Here's how the part is built. I have some questions about the finished solid (model axes, mm). A direction names the side the tool comes from. Round coordinates to 2 decimals unless told otherwise and drop trailing zeros. Loops run counter-clockwise (first coordinate to the right, second up) from the corner with the lowest first, then second, coordinate; pieces in that order, holes last. Notation, with made-up numbers: M -12,40.25 L 38,40.25 A19 ccw 38,50.25 Z; hole C 74.5,-20.5 d2. An arc over 180 degrees is marked long. Write each question's results on one line, items separated by ' | '. Start each with the question number.
```python
from build123d import *

# Parameters (mm, degrees)
SKETCH1_R      = 1.75
EXTRUDE1_DEPTH = 3.15
CHAMFER1_SIZE  = 1.5
EXTRUDE2_START = 1.35
EXTRUDE2_DEPTH = 1.35
EXTRUDE3_DEPTH = 13.7
EXTRUDE4_DEPTH = 3
SKETCH5_W      = 4.8
SKETCH5_H      = 0.7
EXTRUDE5_DEPTH = 6.25
CHAMFER2_SIZE  = 1
EXTRUDE6_DEPTH = 17
FILLET1_R      = 0.5
SKETCH7_W      = 2
SKETCH7_H      = 4
EXTRUDE7_DEPTH = 14
SKETCH8_W      = 2
SKETCH8_H      = 4
EXTRUDE8_DEPTH = 16.5
CHAMFER3_SIZE  = 0.75


with BuildPart() as part:
    # Sketch1 → Extrude1 (new body)
    with BuildSketch(Plane.XY):
        with BuildLine():
            Line((-12.75, 11.25), (12.75, 11.25))
            ThreePointArc((12.75, 11.25), (13.556623081, 11.116296517), (14.276967509, 10.729487365))
            Line((14.276967509, 10.729487365), (23.053935018, 3.958974729))
            ThreePointArc((23.053935018, 3.958974729), (25, 0), (23.053935018, -3.958974729))
            Line((23.053935018, -3.958974729), (14.276967509, -10.729487365))
            ThreePointArc((14.276967509, -10.729487365), (13.556623081, -11.116296517), (12.75, -11.25))
            Line((12.75, -11.25), (-12.75, -11.25))
            ThreePointArc((-12.75, -11.25), (-13.556623081, -11.116296517), (-14.276967509, -10.729487365))
            Line((-14.276967509, -10.729487365), (-23.053935018, -3.958974729))
            ThreePointArc((-23.053935018, -3.958974729), (-25, 0), (-23.053935018, 3.958974729))
            Line((-23.053935018, 3.958974729), (-14.276967509, 10.729487365))
            ThreePointArc((-14.276967509, 10.729487365), (-13.556623081, 11.116296517), (-12.75, 11.25))
        make_face()
        with Locations((-20, 0)):
            Circle(SKETCH1_R, mode=Mode.SUBTRACT)
        with Locations((20, 0)):
            Circle(SKETCH1_R, mode=Mode.SUBTRACT)
    extrude(amount=EXTRUDE1_DEPTH)

    # Chamfer1
    chamfer1_edges = [part.edges().sort_by_distance(p)[0] for p in [
        (-21.75, 0, 0),
        (18.25, 0, 0),
    ]]
    chamfer(chamfer1_edges, length=CHAMFER1_SIZE)

    # Sketch2 → Extrude2 (add)
    with BuildSketch(Plane(origin=(0, 0, 0), x_dir=(-1, 0, 0), z_dir=(0, 0, -1)).offset(EXTRUDE2_START)):
        with BuildLine():
            Line((-12.75, 11.25), (12.75, 11.25))
            ThreePointArc((12.75, 11.25), (14.517766953, 10.517766953), (15.25, 8.75))
            Line((15.25, 8.75), (15.25, -8.75))
            ThreePointArc((15.25, -8.75), (14.517766953, -10.517766953), (12.75, -11.25))
            Line((12.75, -11.25), (-12.75, -11.25))
            ThreePointArc((-12.75, -11.25), (-14.517766953, -10.517766953), (-15.25, -8.75))
            Line((-15.25, -8.75), (-15.25, 8.75))
            ThreePointArc((-15.25, 8.75), (-14.517766953, 10.517766953), (-12.75, 11.25))
        make_face()
    extrude(amount=-EXTRUDE2_DEPTH)

    # Sketch3 → Extrude3 (add)
    with BuildSketch(Plane.XY.offset(3.15)):
        with BuildLine():
            Line((-7.75, 9.4), (7.75, 9.4))
            Line((7.75, 9.4), (13.25, 3.9))
            Line((13.25, 3.9), (13.25, -5.4))
            ThreePointArc((13.25, -5.4), (12.078427125, -8.228427125), (9.25, -9.4))
            Line((9.25, -9.4), (-9.25, -9.4))
            ThreePointArc((-9.25, -9.4), (-12.078427125, -8.228427125), (-13.25, -5.4))
            Line((-13.25, -5.4), (-13.25, 3.9))
            Line((-13.25, 3.9), (-7.75, 9.4))
        make_face()
    extrude(amount=EXTRUDE3_DEPTH)

    # Sketch4 → Extrude4 (add)
    with BuildSketch(Plane.XY.offset(16.85)):
        Polygon((-10.5, 1.25), (-3.5, 1.25), (-3.5, 5.4), (3.5, 5.4), (3.5, 1.25), (10.5, 1.25), (10.5, -5.4), (3.5, -5.4), (3.5, -1.25), (-3.5, -1.25), (-3.5, -5.4), (-10.5, -5.4), align=None)
    extrude(amount=EXTRUDE4_DEPTH)

    # Sketch5 → Extrude5 (add)
    with BuildSketch(Plane.XY.offset(19.85)):
        with Locations((0, 3.55)):
            Rectangle(SKETCH5_W, SKETCH5_H)
        with Locations((7, -3.55)):
            Rectangle(SKETCH5_W, SKETCH5_H)
        with Locations((-7, -3.55)):
            Rectangle(SKETCH5_W, SKETCH5_H)
    extrude(amount=EXTRUDE5_DEPTH)

    # Chamfer2
    chamfer2_edges = [part.edges().sort_by_distance(p)[0] for p in [
        (-2.4, 3.55, 26.1),
        (2.4, 3.55, 26.1),
        (4.6, -3.55, 26.1),
        (9.4, -3.55, 26.1),
        (-9.4, -3.55, 26.1),
        (-4.6, -3.55, 26.1),
    ]]
    chamfer(chamfer2_edges, length=CHAMFER2_SIZE)

    # Sketch6 → Extrude6 (cut)
    with BuildSketch(Plane(origin=(0, 0, -1.35), x_dir=(-1, 0, 0), z_dir=(0, 0, -1))):
        with BuildLine():
            Line((-6.7, 7.85), (6.7, 7.85))
            Line((6.7, 7.85), (12.2, 2.35))
            Line((12.2, 2.35), (12.2, -5.35))
            ThreePointArc((12.2, -5.35), (11.467766953, -7.117766953), (9.7, -7.85))
            Line((9.7, -7.85), (-9.7, -7.85))
            ThreePointArc((-9.7, -7.85), (-11.467766953, -7.117766953), (-12.2, -5.35))
            Line((-12.2, -5.35), (-12.2, 2.35))
            Line((-12.2, 2.35), (-6.7, 7.85))
        make_face()
    extrude(amount=-EXTRUDE6_DEPTH, mode=Mode.SUBTRACT)

    # Fillet1
    fillet1_edges = [part.edges().sort_by_distance(p)[0] for p in [
        (9.45, 5.1, -1.35),
        (12.2, -1.5, -1.35),
        (11.467766953, -7.117766953, -1.35),
        (0, -7.85, -1.35),
        (-11.467766953, -7.117766953, -1.35),
        (-12.2, -1.5, -1.35),
        (-9.45, 5.1, -1.35),
        (0, 7.85, -1.35),
    ]]
    fillet(fillet1_edges, radius=FILLET1_R)

    # Sketch7 → Extrude7 (add)
    with BuildSketch(Plane(origin=(0, 0, 15.65), x_dir=(-1, 0, 0), z_dir=(0, 0, -1))):
        with Locations((-7, -2)):
            Rectangle(SKETCH7_W, SKETCH7_H)
        with Locations((7, -2)):
            Rectangle(SKETCH7_W, SKETCH7_H)
    extrude(amount=EXTRUDE7_DEPTH)

    # Sketch8 → Extrude8 (add)
    with BuildSketch(Plane(origin=(0, 0, 15.65), x_dir=(-1, 0, 0), z_dir=(0, 0, -1))):
        with Locations((0, 2)):
            Rectangle(SKETCH8_W, SKETCH8_H)
    extrude(amount=EXTRUDE8_DEPTH)

    # Chamfer3
    chamfer3_edges = [part.edges().sort_by_distance(p)[0] for p in [
        (8, -2, 1.65),
        (7, -4, 1.65),
        (6, -2, 1.65),
        (7, 0, 1.65),
        (-6, -2, 1.65),
        (-7, -4, 1.65),
        (-8, -2, 1.65),
        (-7, 0, 1.65),
        (1, 2, -0.85),
        (0, 0, -0.85),
        (-1, 2, -0.85),
        (0, 4, -0.85),
    ]]
    chamfer(chamfer3_edges, length=CHAMFER3_SIZE)


solid = part.part
```
1. I want a section at C-C on x = -20. List the corners of the cut face in (y, z) for me, plus the area to 3 significant figures.
2. I want a section at A-A on z = 6. List the corners of the cut face in (x, y) for me, plus the area to 3 significant figures.
3. Which directions (+Z, -Z, +X, -X, +Y, -Y) give clear straight access to the entire face, cutting with the end or side of a thin tool? Please do faces 5 (the face through (-9.6, 5.17, -1.21)), 6 (the face through (-5.1, -3.6, 25.6)), 7 (the face through (10.5, -2, 18)), 8 (the face through (0, 10, 3.15)), 9 (the face through (-7, 1.25, 18)).
4. For pin 1 (0.9 mm diameter, centred on x = 7, z = 18, fed in from +Y); pin 2 (1.5 mm diameter, centred on y = -5.5, z = 2.5, fed in from -X); pin 3 (2.5 mm diameter, centred on x = 6.5, z = 23, fed in from -Y), each with a flat end and sliding along its axis, tell me the tip position at first contact or that it passes through.
5. I want a section at B-B on z = 23.5. List the corners of the cut face in (x, y) for me.
6. If we mould it in two halves opening along Y, with no side actions, what happens to faces 1 (the face through (8, -2, 9)), 2 (the face through (7, -4, 9)), 3 (the face through (0, 10, -1.35)), 4 (the face through (0, -11.25, 1))? For each: released by +Y, released by -Y, zero draft, split by the parting line, or undercut.
7. I need wall thicknesses on line 1 along X through (y, z) = (1, 6); line 2 along X through (y, z) = (-4.5, 15.5); line 3 along X through (y, z) = (3.75, 8). Which ranges of each line are inside material? Lowest first, please.
Outcome:
1) outline: M -6.31,0 L -3.25,0 L -1.75,1.5 L -1.75,3.15 L -6.31,3.15 Z; M 1.75,1.5 L 3.25,0 L 6.31,0 L 6.31,3.15 L 1.75,3.15 Z | area: 26.5 mm2
2) outline: M -13.25,-5.4 A4 ccw -9.25,-9.4 L 9.25,-9.4 A4 ccw 13.25,-5.4 L 13.25,3.9 L 7.75,9.4 L -7.75,9.4 L -13.25,3.9 Z; M -8,-4 L -6,-4 L -6,0 L -8,0 Z; M -1,0 L 1,0 L 1,4 L -1,4 Z; M 6,-4 L 8,-4 L 8,0 L 6,0 Z; hole M -12.2,-5.35 A2.5 ccw -9.7,-7.85 L 9.7,-7.85 A2.5 ccw 12.2,-5.35 L 12.2,2.35 L 6.7,7.85 L -6.7,7.85 L -12.2,2.35 Z | area: 135 mm2
3) face 5: -Z | face 6: +Z, +Y, -Y | face 7: +Z, +X, +Y, -Y | face 8: +Z | face 9: +Z, -X, +Y
4) pin 1: y = 1.25 | pin 2: x = -22.03 | pin 3: y = -3.9
5) outline: M -9.4,-3.9 L -4.6,-3.9 L -4.6,-3.2 L -9.4,-3.2 Z; M -2.4,3.2 L 2.4,3.2 L 2.4,3.9 L -2.4,3.9 Z; M 4.6,-3.9 L 9.4,-3.9 L 9.4,-3.2 L 4.6,-3.2 Z
6) face 1: undercut | face 2: undercut | face 3: zero draft | face 4: released by -Y
7) line 1: -13.25 to -12.2, -1 to 1, 12.2 to 13.25 | line 2: -13.25 to -12.2, 12.2 to 13.25 | line 3: -13.25 to -10.8, -1 to 1, 10.8 to 13.25
